```python
from build123d import *

# Parameters (mm, degrees)
SKETCH1_R               = 3.5
SKETCH1_R_2             = 1.65
SKETCH1_W               = 10
SKETCH1_H               = 4
BOSS_EXTRUDE1_DEPTH     = 30
FILLET1_R               = 3
FILLET2_R               = 3
CUT_EXTRUDE1_DEPTH      = 15
CUT_EXTRUDE2_DEPTH      = 7
CUT_EXTRUDE2_DEPTH_BACK = 15
SKETCH3_R               = 1.65
CUT_EXTRUDE3_DEPTH      = 15
CUT_EXTRUDE3_DEPTH_BACK = 1.5
SKETCH4_R               = 3.5


with BuildPart() as part:
    # Sketch1 → Boss-Extrude1 (new body)
    # profile 1 of 3: a face of its own
    with BuildSketch(Plane.XY):
        with Locations((-2.1, 8.4)):
            Circle(SKETCH1_R)
        with Locations((-2.1, 8.4)):
            Circle(SKETCH1_R_2, mode=Mode.SUBTRACT)
    # profile 2 of 3: a face of its own
    with BuildSketch(Plane.XY):
        with BuildLine():
            Line((0, 5.6), (0, 4))
            Line((0, 4), (1.4, 4))
            Line((1.4, 4), (1.4, 8.4))
            ThreePointArc((1.4, 8.4), (1.030495168, 6.834752416), (0, 5.6))
        make_face()
    # profile 3 of 3: a face of its own
    with BuildSketch(Plane.XY):
        with Locations((5, 2)):
            Rectangle(SKETCH1_W, SKETCH1_H)
    extrude(amount=-BOSS_EXTRUDE1_DEPTH)

    # Fillet1
    fillet1_edges = [part.edges().sort_by_distance(p)[0] for p in [
        (1.4, 4, -15),
    ]]
    fillet(fillet1_edges, radius=FILLET1_R)

    # Fillet2
    fillet2_edges = [part.edges().sort_by_distance(p)[0] for p in [
        (0, 5.6, -15),
    ]]
    fillet(fillet2_edges, radius=FILLET2_R)

    # Sketch2 → Cut-Extrude1 (cut)
    with BuildSketch(Plane(origin=(0, 0, -30), x_dir=(-1, 0, 0), z_dir=(0, 0, -1))):
        Polygon((-4.4, 4), (0, 4), (0, 0), (6.883389495, 0), (6.883389495, 4), (6.883389495, 12.878531322), (-4.4, 12.878531322), align=None)
    extrude(amount=-CUT_EXTRUDE1_DEPTH, mode=Mode.SUBTRACT)

    # Sketch3 → Cut-Extrude2 (cut, two sides: drawn at the far end of the back side and taken through both)
    with BuildSketch(Plane(origin=(0, 4, 0), x_dir=(1, 0, 0), z_dir=(0, 1, 0)).offset(-CUT_EXTRUDE2_DEPTH_BACK)):
        with Locations(Location((5, 5, 0), (0, 0, 90))):
            Circle(SKETCH3_R)
        with Locations(Location((5, 25, 0), (0, 0, 90))):
            Circle(SKETCH3_R)
    extrude(amount=CUT_EXTRUDE2_DEPTH + CUT_EXTRUDE2_DEPTH_BACK, mode=Mode.SUBTRACT)

    # Sketch4 → Cut-Extrude3 (cut, two sides: drawn at the far end of the back side and taken through both)
    with BuildSketch(Plane(origin=(0, 4, 0), x_dir=(1, 0, 0), z_dir=(0, 1, 0)).offset(-CUT_EXTRUDE3_DEPTH_BACK)):
        with Locations(Location((5, 5, 0), (0, 0, 99.870889606))):
            Circle(SKETCH4_R)
        with Locations(Location((5, 25, 0), (0, 0, 90))):
            Circle(SKETCH4_R)
    extrude(amount=CUT_EXTRUDE3_DEPTH + CUT_EXTRUDE3_DEPTH_BACK, mode=Mode.SUBTRACT)


solid = part.part
```
Can you work these out from the model? Positions are in its coordinate system, mm. A direction names the side the tool comes from. Round coordinates to 2 decimals unless told otherwise and drop trailing zeros. Loops run counter-clockwise (first coordinate to the right, second up) from the corner with the lowest first, then second, coordinate; pieces in that order, holes last. Notation, with made-up numbers: (45, 26.5) -> (86, 26.5) arc R24 ccw to (86, 41.5) -> close; hole circle Ø8 at (-17, 19). An arc over 180 degrees is marked (long way). Answer in a Markdown table with one row per item.
Item 1: Suppose I cut it at B-B, the plane x = -3. List the corners of the cut face in (y, z) for me.
Answer block:
| item | result |
|---|---|
| outline | (5.02, -15) -> (7.02, -15) -> (7.02, 0) -> (5.02, 0) -> close; (9.78, -15) -> (11.78, -15) -> (11.78, 0) -> (9.78, 0) -> close |
Item 2: Suppose I cut it at C-C, the plane z = -9.5. List the corners of the cut face in (x, y) for me, plus the area to 3 significant figures.
Answer block:
| item | result |
|---|---|
| outline | (-2.58, 4.93) arc R3 cw to (0, 1.96) -> (0, 0) -> (10, 0) -> (10, 4) -> (4.4, 4) arc R3 cw to (1.4, 7) -> (1.4, 8.4) arc R3.5 ccw (long way) to start; hole circle Ø3.3 at (-2.1, 8.4) |
| area | 77.5 mm² |
Item 3: On a 3-axis mill with a long thin cutter (end or side, diameter ignored), from which of +Z, -Z, +X, -X, +Y, -Y can I reach the whole of each face in a straight line? I mean faces 4 (the flat face through (5, 2.5, -7)), 5 (the flat face through (0, 2, -18)), 6 (the flat face through (1.4, 8, -7)). Say none if no direction works.
Answer block:
| item | result |
|---|---|
| face 4 | +Y |
| face 5 | -Z, -X, -Y |
| face 6 | +Z, -Z, +X, +Y |
Item 4: If I drill on probe 1 along Y at (x, z) = (8, -4); probe 2 along Y at (x, z) = (-2.1, -8); probe 3 along Y at (x, z) = (-3.25, -9.5), over which ranges is the centre line in solid material (lowest first)?
Answer block:
| item | result |
|---|---|
| probe 1 | 0 to 2.5 |
| probe 2 | 4.82 to 6.75, 10.05 to 11.9 |
| probe 3 | 5.09 to 7.22, 9.58 to 11.71 |
Item 5: Will these pins go through, and if not, where does the flat tip stop? P1, Ø5.5, axis at x = 6.5, z = -26.5, coming from the +Y side; P2, Ø1.1, axis at y = 8, z = -5.5, coming from the +X side; P3, Ø2, axis at x = 5.5, z = -5.5, coming from the +Y side.
Answer block:
| item | result |
|---|---|
| P1 | y = 4 |
| P2 | x = 1.4 |
| P3 | y = 2.5 |
Item 6: Suppose I cut it at A-A, the plane z = -5. List the corners of the cut face in (x, y) for me, plus the area to 3 significant figures.
Answer block:
| item | result |
|---|---|
| outline | (-2.58, 4.93) arc R3 cw to (0, 1.96) -> (0, 0) -> (3.35, 0) -> (3.35, 2.5) -> (1.5, 2.5) -> (1.5, 6.23) arc R3 cw to (1.4, 7) -> (1.4, 8.4) arc R3.5 ccw (long way) to start; (6.65, 0) -> (10, 0) -> (10, 4) -> (8.5, 4) -> (8.5, 2.5) -> (6.65, 2.5) -> close; hole circle Ø3.3 at (-2.1, 8.4) |
| area | 57.1 mm² |
Item 7: Suppose I cut it at D-D, the plane y = 3.25. List the corners of the cut face in (x, z) for me, plus the area to 3 significant figures.
Answer block:
| item | result |
|---|---|
| outline | (-0.29, -15) -> (0, -15) -> (0, -30) -> (10, -30) -> (10, 0) -> (-0.29, 0) -> close; hole circle Ø7 at (5, -25); hole circle Ø7 at (5, -5) |
| area | 227 mm² |
Item 8: We'd pull the mould along Y, two halves only. Please class faces 1 (the cylindrical face through (-0.8, 4, -7.6)), 2 (the flat face through (5, 2, -30)), 3 (the cylindrical face through (-0.576, 7.768, -7.395)): released by +Y, released by -Y, zero draft, split by the parting line, or undercut.
Answer block:
| item | result |
|---|---|
| face 1 | released by -Y |
| face 2 | zero draft |
| face 3 | undercut |
